Check sheet for the modelled part. Datum: model origin and axes. Units: mm. Coordinates: 2 decimals unless noted, no trailing zeros. Write each loop counter-clockwise with the first axis right and the second up, starting at its lowest first coordinate (ties: lowest second). Pieces come first, ordered by that corner, then holes. Notation, with made-up numbers: (66.25, 67.5) -> (94.25, 67.5) arc R12 cw to (94.25, 73.5) -> close; hole circle Ø6 at (-16, 0.25). An arc over 180 degrees is marked (long way). One line per item, written item: value. Start each with the question number.
1) Gauge pin test, flat end, axial feed: P1, Ø3, axis at x = 0, z = 80, coming from the -Y side. Record the tip position at first contact, or that the pin passes through.
2) Sectioned sample at B-B on z = 80. Enter the section's corners in (x, y).
3) Sectioned sample at C-C on y = -2.5. Enter the section's corners in (x, z).
4) Scan lines: line 1 along Z through (x, y) = (0, -1.5); line 2 along Z through (x, y) = (1, -1.5); line 3 along X through (y, z) = (1.5, 81.5). Record each from-to range of solid material in increasing order. Write a range as [from, to].
5) Sectioned sample at A-A on x = 0. Enter the section's corners in (y, z).
```python
from build123d import *

# Parameters (mm, degrees)
F0_W     = 10
F0_H     = 10
F1_DEPTH = 100
F3_D     = 3.4


with BuildPart() as f1:
    # F0 (on Top) → F1 (new body)
    with BuildSketch(Plane.XY):
        Rectangle(F0_W, F0_H)
    extrude(amount=F1_DEPTH)

    # F3 (through all)
    with Locations(Plane.XZ.offset(5)):
        with Locations((0, 80), (0, 20)):
            Hole(F3_D / 2)


solid = f1.part
```
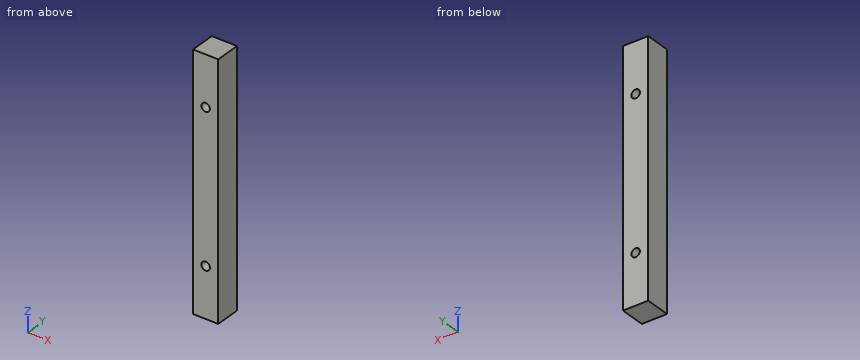
Answers:
1. P1: passes through
2. outline: (-5, -5) -> (-1.7, -5) -> (-1.7, 5) -> (-5, 5) -> close; (1.7, -5) -> (5, -5) -> (5, 5) -> (1.7, 5) -> close
3. outline: (-5, 0) -> (5, 0) -> (5, 100) -> (-5, 100) -> close; hole circle Ø3.4 at (0, 20); hole circle Ø3.4 at (0, 80)
4. line 1: z = [0, 18.3], [21.7, 78.3], [81.7, 100]
4. line 2: z = [0, 18.63], [21.37, 78.63], [81.37, 100]
4. line 3: x = [-5, -0.8], [0.8, 5]
5. outline: (-5, 0) -> (5, 0) -> (5, 18.3) -> (-5, 18.3) -> close; (-5, 21.7) -> (5, 21.7) -> (5, 78.3) -> (-5, 78.3) -> close; (-5, 81.7) -> (5, 81.7) -> (5, 100) -> (-5, 100) -> close
